```python
from build123d import *

# Parameters (mm, degrees)
ODEBRAT_VYSUNUT_M1_DEPTH = 8
SKICA3_R                 = 1.5
ODEBRAT_VYSUNUT_M2_DEPTH = 2


with BuildPart() as part:
    # Skica1 → Rotovat1 (revolve)
    with BuildSketch(Plane.XY):
        with BuildLine():
            Line((0, 0), (3.25, 0))
            Line((3.25, 0), (3.25, 2))
            Line((3.25, 2), (12.2, 2))
            Line((12.2, 2), (12.2, 31.3))
            ThreePointArc((12.2, 31.3), (11.760660172, 32.360660172), (10.7, 32.8))
            Line((10.7, 32.8), (12.5, 32.8))
            Line((12.5, 32.8), (12.5, 53.8))
            Line((12.5, 53.8), (3.5, 53.8))
            Line((3.5, 53.8), (3.5, 56.3))
            Line((3.5, 56.3), (2, 56.3))
            Line((2, 56.3), (2, 64.8))
            Line((2, 64.8), (0, 64.8))
            Line((0, 64.8), (0, 0))
        make_face()
    revolve(axis=Axis((0, 0, 0), (0, 1, 0)))

    # Skica2 → Odebrat vysunutím1 (cut)
    with BuildSketch(Plane(origin=(0, 64.8, 0), x_dir=(1, 0, 0), z_dir=(0, 1, 0))):
        with BuildLine():
            Line((1.5, 1.322875656), (1.5, -1.322875656))
            ThreePointArc((1.5, -1.322875656), (2, 0), (1.5, 1.322875656))
        make_face()
    extrude(amount=-ODEBRAT_VYSUNUT_M1_DEPTH, mode=Mode.SUBTRACT)

    # Skica3 → Odebrat vysunutím2 (cut)
    with BuildSketch(Plane(origin=(0, 53.8, 0), x_dir=(1, 0, 0), z_dir=(0, 1, 0))):
        with Locations((8.5, 0)):
            Circle(SKICA3_R)
        with Locations((-8.5, 0)):
            Circle(SKICA3_R)
    extrude(amount=-ODEBRAT_VYSUNUT_M2_DEPTH, mode=Mode.SUBTRACT)


solid = part.part
```
The listing builds one solid part. Answer for the finished solid, in the listing's coordinates (mm). A direction names the side the tool comes from. Give positions to 0.01 mm unless a question says otherwise; leave off trailing zeros. Order: outer loops, then holes, each group sorted by start corner. A loop starts at its lowest first (then second) coordinate and runs counter-clockwise, first axis right, second up.
Item 1: The part is cut by section D-D, the plane y = 10. Give the vertices of the cut face in (x, z), and give its area (3 significant figures).
From the geometry:
outline: circle Ø24.4 at (0, 0)
area: 468 mm2
Item 2: The part is cut by section B-B, the plane x = 0. Give the vertices of the cut face in (y, z).
From the geometry:
outline: (0, -3.25) - (2, -3.25) - (2, -12.2) - (31.3, -12.2) arc R1.5 ccw to (32.8, -10.7) - (32.8, -12.5) - (53.8, -12.5) - (53.8, -3.5) - (56.3, -3.5) - (56.3, -2) - (64.8, -2) - (64.8, 2) - (56.3, 2) - (56.3, 3.5) - (53.8, 3.5) - (53.8, 12.5) - (32.8, 12.5) - (32.8, 10.7) arc R1.5 ccw to (31.3, 12.2) - (2, 12.2) - (2, 3.25) - (0, 3.25) - close
Item 3: Which of the six approach directions +Z, -Z, +X, -X, +Y, -Y give full straight-line access (tool end or side, diameter ignored) to faces 1 (the face through (8, 51.8, 0)), 2 (the face through (1.5, 61, 0)), 3 (the face through (-2.579, 1.014, 1.978))?
From the geometry:
face 1: +Y
face 2: +Z, -Z, +X, +Y
face 3: -Y
Item 4: Given pin 1 Ø1.8 at (x, z) = (8.5, 0) entering from -Y; pin 2 Ø5 at (x, y) = (0, 8) entering from -Z; pin 3 Ø2 at (x, y) = (-5.5, 36.5) entering from +Z; pin 4 Ø6 at (x, z) = (-3, -0.5) entering from -Y, each flat-ended and moving along its own axis, determine where each tip first touches the part or whether it passes through.
From the geometry:
pin 1: stops at y = 2
pin 2: stops at z = -12.2
pin 3: stops at z = 11.66
pin 4: stops at y = 0
Item 5: Find the intervals of material crossed by probe 1 along X at (y, z) = (52.35, 0); probe 2 along Z at (x, y) = (0, 31); probe 3 along Y at (x, z) = (-2.75, -9.75), in increasing order.
From the geometry:
probe 1: x = -12.5 to -10, -7 to 7, 10 to 12.5
probe 2: z = -12.2 to 12.2
probe 3: y = 2 to 53.8
Item 6: The part is cut by section C-C, the plane y = 52.5. Give the vertices of the cut face in (x, z).
From the geometry:
outline: circle Ø25 at (0, 0); hole circle Ø3 at (-8.5, 0); hole circle Ø3 at (8.5, 0)
